The listing builds one solid part. Answer for the finished solid, in the listing's coordinates (mm). Give positions to 0.01 mm unless a question says otherwise; leave off trailing zeros. Loops run counter-clockwise (first coordinate to the right, second up) from the corner with the lowest first, then second, coordinate; pieces in that order, holes last. Notation, with made-up numbers: (-18, 4.5) -> (15, 4.5) arc R26 cw to (15, 41.5) -> close; hole circle Ø11 at (71, -30). An arc over 180 degrees is marked (long way). One line per question, with ' | ' between items. Start each with the question number.
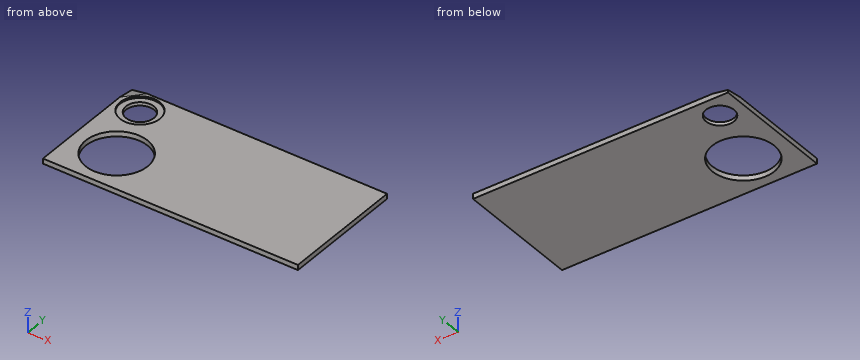
Autodesk Inventor part; units mm, degrees
ref_plane "РабПлоскость9" through (0, 290, -6) normal (0.1626, -0.1464, -0.9758) x (0.9864, 0, 0.1644)
ref_plane "YZ Plane" through (0, 0, 0) normal (1, 0, 0) x (0, 1, 0)
ref_plane "XZ Plane" through (0, 0, 0) normal (0, 1, 0) x (-1, 0, 0)
sketch "Front0" plane through (0, 0, 0) normal (0, 0, 1) x (1, 0, 0)
  line L0 (0, 0) -> (600, 0)
  line L1 (600, 0) -> (600, 290)
  line L2 (600, 290) -> (0, 290)
  line L3 (0, 290) -> (0, 0)
  circle A0 centre (104, 96) radius 73
  circle A1 centre (104, 96) radius 91
  circle A2 centre (57, 237) radius 47
  circle A3 centre (57, 237) radius 33
  line L4 (36, 290) -> (0, 250)
  line L5 (196, 290) -> (196, 0) construction
  point P0 (47.17, 0)
  point P1 (0, 87)
  dimension "d0" = 600
  dimension "d1" = 290
  dimension "d2" = 146
  dimension "d3" = 182
  dimension "d4" = 94
  dimension "d5" = 66
  dimension "d17" = 96
  dimension "d36" = 104
  dimension "d37" = 57
  dimension "d38" = 53
  dimension "d40" = 92
  dimension "d24" = 146
  dimension "d25" = 182
extrude "Выдавливание2" add sketch "Front0" against normal blind 12 contours L3 L4 L2 L1 L0 | L3 L2 L4 | A1 | A2
ref_plane "РабПлоскость9" through (0, 290, -6) normal (0.1626, -0.1464, -0.9758) x (0.9864, 0, 0.1644)
split "Разделение5" plane through (0, 290, -6) removes the side toward (-0.1626, 0.1464, 0.9758)
extrude "Выдавливание7" cut sketch "Front0" against normal blind 4 contours A2
properties part number "Front_L"
1. The part is cut by section B-B (x = 57). Write down the section's boundary in (y, z), plus the area to 3 significant figures.
2. Straight lines are drawn through the part: L1, parallel to Y at x = 104, z = -6.75; L2, parallel to Y at x = 57, z = -8.25; L3, parallel to Y at x = 158, z = -1.5. For each, find the intervals that lie inside material, in ascending order.
3. The part is cut by section A-A (y = 237). Write down the section's boundary in (x, z).
4. The part is cut by section D-D (y = 45.5). Write down the section's boundary in (x, z), plus the area to 3 significant figures.
5. The part is cut by section C-C (y = 96). Write down the section's boundary in (x, z).
Check sheet entries:
1) outline: (0, -12) -> (40.14, -12) -> (40.14, 0) -> (0, 0) -> close; (151.86, -12) -> (204, -12) -> (204, -4) -> (190, -4) -> (190, 0) -> (151.86, 0) -> close; (270, -12) -> (290, -12) -> (290, 0) -> (284, 0) -> (284, -4) -> (270, -4) -> close | area: 1,240 mm^2
2) L1: y = 0 to 23, 169 to 290 | L2: y = 0 to 40.14, 151.86 to 204, 270 to 290 | L3: y = 0 to 46.88, 145.12 to 290
3) outline: (0, -12) -> (24, -12) -> (24, -4) -> (10, -4) -> (10, 0) -> (0, 0) -> close; (90, -12) -> (600, -12) -> (600, 0) -> (104, 0) -> (104, -4) -> (90, -4) -> close
4) outline: (0, -12) -> (51.29, -12) -> (51.29, 0) -> (0, 0) -> close; (156.71, -12) -> (600, -12) -> (600, 0) -> (156.71, 0) -> close | area: 5,930 mm^2
5) outline: (0, -12) -> (31, -12) -> (31, 0) -> (0, 0) -> close; (177, -12) -> (600, -12) -> (600, 0) -> (177, 0) -> close
